Could you check a few things on this model? Use its own coordinates, in mm. A direction names the side the tool comes from. Coordinates: 2 decimals unless noted, no trailing zeros. Write each loop counter-clockwise with the first axis right and the second up, starting at its lowest first coordinate (ties: lowest second). Pieces come first, ordered by that corner, then holes. Notation, with made-up numbers: M 36,59 L 91,59 A25 ccw 91,72 Z; hole C 30.5,63.25 d1. An arc over 180 degrees is marked long. Write item = value, one per line.
```python
from build123d import *

# Parameters (mm, degrees)
F0_W     = 55
F0_H     = 55
F1_DEPTH = 35
F2_W     = 45
F2_H     = 45
F3_DEPTH = 30
F4_R     = 3


with BuildPart() as f1:
    # F0 (on Top) → F1 (new body)
    with BuildSketch(Plane.XY):
        with Locations((-35.2636, 31.343543)):
            Rectangle(F0_W, F0_H)
    extrude(amount=F1_DEPTH)

    # F2 (on face) → F3 (cut)
    with BuildSketch(Plane(origin=(0, 0, 0), x_dir=(1, 0, 0), z_dir=(0, 0, -1))):
        with Locations((-35.2636, -31.343543)):
            Rectangle(F2_W, F2_H)
    extrude(amount=-F3_DEPTH, mode=Mode.SUBTRACT)

    # F4
    f4_edges = [f1.edges().sort_by_distance(p)[0] for p in [
        (-62.7636, 31.343543, 35),
        (-35.2636, 3.843543, 35),
        (-62.7636, 3.843543, 17.5),
        (-7.7636, 31.343543, 35),
        (-35.2636, 58.843543, 35),
        (-62.7636, 58.843543, 17.5),
        (-7.7636, 58.843543, 17.5),
        (-7.7636, 3.843543, 17.5),
    ]]
    fillet(f4_edges, radius=F4_R)


solid = f1.part
```
Item 1: Imagine slicing it at A-A (z = 27.5). Write out the boundary of the cut face in (x, y).
Numbers:
outline = M -62.76,6.84 A3 ccw -59.76,3.84 L -10.76,3.84 A3 ccw -7.76,6.84 L -7.76,55.84 A3 ccw -10.76,58.84 L -59.76,58.84 A3 ccw -62.76,55.84 Z; hole M -57.76,8.84 L -12.76,8.84 L -12.76,53.84 L -57.76,53.84 Z
Item 2: If we mould it in two halves opening along Y, with no side actions, what happens to faces 1 (the face through (-36, 3.844, 16)), 2 (the face through (-36, 53.844, 15)), 3 (the face through (-7.764, 31, 16))? For each: pulls with the +Y half, pulls with the -Y half, needs draft (parallel to the pull), parting line crosses it, or undercut.
Numbers:
face_1 = pulls with the -Y half
face_2 = undercut
face_3 = needs draft
Item 3: Imagine slicing it at C-C (x = -20.5). Write out the boundary of the cut face in (y, z).
Numbers:
outline = M 3.84,0 L 8.84,0 L 8.84,30 L 53.84,30 L 53.84,0 L 58.84,0 L 58.84,32 A3 ccw 55.84,35 L 6.84,35 A3 ccw 3.84,32 Z
Item 4: For faces 4 (the face through (-36, 31, 30)), 5 (the face through (-60, 32, 0)), which set-ups out of +Z, -Z, +X, -X, +Y, -Y let a thin tool reach every point of the face, with its end or its side?
Numbers:
face_4 = -Z
face_5 = -Z, +X, -X, +Y, -Y
Item 5: Imagine slicing it at B-B (y = 50). Write out the boundary of the cut face in (x, z).
Numbers:
outline = M -62.76,0 L -57.76,0 L -57.76,30 L -12.76,30 L -12.76,0 L -7.76,0 L -7.76,32 A3 ccw -10.76,35 L -59.76,35 A3 ccw -62.76,32 Z
Item 6: If I drill on line 1 along Y through (x, z) = (-24, 2.5); line 2 along X through (y, z) = (20, 9); line 3 along Z through (x, y) = (-26, 41.5), over which ranges is the centre line in solid material (lowest first)?
Numbers:
line_1 = 3.84 to 8.84, 53.84 to 58.84
line_2 = -62.76 to -57.76, -12.76 to -7.76
line_3 = 30 to 35
Item 7: I'm going to push a flat-ended pin straight in: P1, Ø1.5, axis at x = -15.5, y = 16.5, coming from the -Z side. Where does the tip first touch, or does it pass through?
Numbers:
P1 = 30
